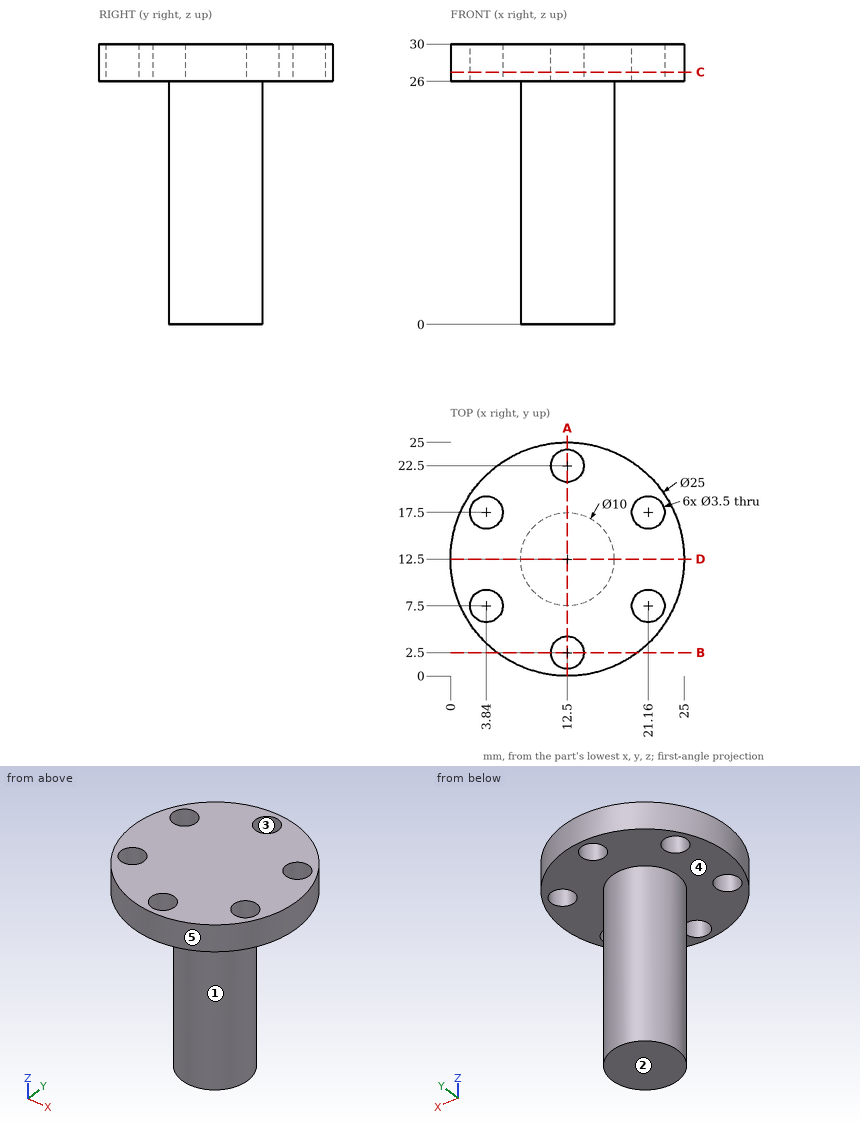
Drawing for the job (mm, zero at the part's lowest x, y, z). A direction names the side the tool comes from. Round coordinates to 2 decimals unless told otherwise and drop trailing zeros. Write each loop counter-clockwise with the first axis right and the second up, starting at its lowest first coordinate (ties: lowest second). Pieces come first, ordered by that corner, then holes. Notation, with made-up numbers: (49.25, 48.25) - (68.25, 48.25) arc R13 cw to (68.25, 52.25) - close; hole circle Ø9 at (-21.75, 20.5). An arc over 180 degrees is marked (long way). Return JSON: item names as keys, results as strings. Group by question number.
Item 1: Flat gauge pins, fed straight in: pin 1 Ø2 at (x, z) = (4, 24) entering from +Y; pin 2 Ø2 at (x, z) = (9, 14.5) entering from +Y; pin 3 Ø8 at (x, z) = (14, 18) entering from +Y; pin 4 Ø6 at (x, z) = (14, 6) entering from -Y. Where does each tip first touch, or does it go through?
Item 2: Band-saw the part on C-C on z = 27. List the corners of the cut face in (x, y), plus the area to 3 significant figures.
Item 3: Band-saw the part on D-D on y = 12.5. List the corners of the cut face in (x, z).
Item 4: Mould opens along X. For the marked faces 3, 4 and 5 say: +X half, -X half, draft (parallel to the pull), parting line (faces both ways), or undercut.
Item 5: Band-saw the part on B-B on y = 2.5. List the corners of the cut face in (x, z).
Item 6: Band-saw the part on A-A on x = 12.5. List the corners of the cut face in (y, z).
Item 7: Probe probe 1 along Y at (x, z) = (12.5, 27.1); probe 2 along Y at (x, z) = (22.5, 26.5) (1 decimal); probe 3 along X at (y, z) = (6.5, 28) (1 decimal). List the from-to ranges inside material, lowest first.
Item 8: 3-axis set-ups, long thin cutter, end or side, ignore diameter. For the marked faces 1 and 2: which of +Z, -Z, +X, -X, +Y, -Y reach the whole face in a straight line?
Resolved:
{
 "1": {"pin 1": "passes through", "pin 2": "stops at y = 16.83", "pin 3": "stops at y = 17.5", "pin 4": "stops at y = 7.5"},
 "2": {"outline": "circle Ø25 at (12.5, 12.5); hole circle Ø3.5 at (3.84, 7.5); hole circle Ø3.5 at (3.84, 17.5); hole circle Ø3.5 at (12.5, 2.5); hole circle Ø3.5 at (12.5, 22.5); hole circle Ø3.5 at (21.16, 7.5); hole circle Ø3.5 at (21.16, 17.5)", "area": "433 mm²"},
 "3": {"outline": "(0, 26) - (7.5, 26) - (7.5, 0) - (17.5, 0) - (17.5, 26) - (25, 26) - (25, 30) - (0, 30) - close"},
 "4": {"face 3": "undercut", "face 4": "draft", "face 5": "parting line"},
 "5": {"outline": "(5, 26) - (10.75, 26) - (10.75, 30) - (5, 30) - close; (14.25, 26) - (20, 26) - (20, 30) - (14.25, 30) - close"},
 "6": {"outline": "(0, 26) - (0.75, 26) - (0.75, 30) - (0, 30) - close; (4.25, 26) - (7.5, 26) - (7.5, 0) - (17.5, 0) - (17.5, 26) - (20.75, 26) - (20.75, 30) - (4.25, 30) - close; (24.25, 26) - (25, 26) - (25, 30) - (24.25, 30) - close"},
 "7": {"probe 1": "y = 0 to 0.75, 4.25 to 20.75, 24.25 to 25", "probe 2": "y = 5 to 6.4, 8.6 to 16.4, 18.6 to 20", "probe 3": "x = 1.5 to 2.4, 5.3 to 19.7, 22.6 to 23.5"},
 "8": {"face 1": "-Z", "face 2": "-Z, +X, -X, +Y, -Y"}
}
